Here's how the part is built. I have some questions about the finished solid (model axes, mm). Face numbers are marked on the shaded views. A direction names the side the tool comes from. Give positions to 0.01 mm unless a question says otherwise; leave off trailing zeros. Loops run counter-clockwise (first coordinate to the right, second up) from the corner with the lowest first, then second, coordinate; pieces in that order, holes last.
Q1. If we section it at D-D (z = -11): Please give me the cut outline in (x, y).
Q2. If we section it at B-B (z = 16.5): Please give me the cut outline in (x, y).
Q3. If we section it at A-A (y = 2.8): Please give me the cut outline in (x, z).
Q4. I need wall thicknesses on line 1 (Z direction, x = -33.2, y = 1.7); line 2 (X direction, y = 2.9, z = 0); line 3 (Y direction, x = 14, z = -13). Which ranges of each line are inside material? Lowest first, please.
Q5. If we section it at C-C (x = 8.5): Please give me the cut outline in (y, z).
Q6. We'd pull the mould along X, two halves only. Please class the marked faces 1 and 2: +X half, -X half, draft (parallel to the pull), parting line (faces both ways), or undercut.
Q7. For the marked faces 3 and 4, which set-ups out of +Z, -Z, +X, -X, +Y, -Y let a thin tool reach every point of the face, with its end or its side?
Q8. Will these pins go through, and if not, where does the flat tip stop? P1, Ø0.7, axis at x = -33.2, z = 23, coming from the +Y side; P2, Ø1.4, axis at x = -33.2, z = -24.7, coming from the -Y side; P3, Ø1.3, axis at x = 29.4, z = 19.4, coming from the +Y side (3 decimals).
from build123d import *

# Parameters (mm, degrees)
SKETCH1_W                         = 71
SKETCH1_H                         = 54
BOSS_EXTRUDE1_DEPTH               = 4.15
CUT_EXTRUDE1_DEPTH                = 2
SKETCH4_R                         = 7.5
BOSS_EXTRUDE3_DEPTH               = 2
SKETCH5_R                         = 24
BOSS_EXTRUDE4_DEPTH               = 0.15
M1_4X0_3_TAPPED_HOLE1_D           = 1.1
M1_4X0_3_TAPPED_HOLE1_CSINK_D     = 1.45
M1_4X0_3_TAPPED_HOLE1_CSINK_ANGLE = 90
FILLET1_R                         = 2


with BuildPart() as part:
    # Sketch1 → Boss-Extrude1 (new body)
    with BuildSketch(Plane(origin=(0, 0, 0), x_dir=(1, 0, 0), z_dir=(0, 1, 0))):
        Rectangle(SKETCH1_W, SKETCH1_H)
    extrude(amount=BOSS_EXTRUDE1_DEPTH)

    # Sketch3 → Cut-Extrude1 (cut)
    with BuildSketch(Plane(origin=(0, 4.15, 0), x_dir=(1, 0, 0), z_dir=(0, 1, 0))):
        with BuildLine():
            Line((-6.5, 20), (-33.5, 20))
            Line((-33.5, 20), (-33.5, -19))
            Line((-33.5, -19), (-7.748076809, -19))
            ThreePointArc((-7.748076809, -19), (33.487208249, -0.799639875), (-6.5, 20))
        make_face()
    extrude(amount=-CUT_EXTRUDE1_DEPTH, mode=Mode.SUBTRACT)

    # Sketch4 → Boss-Extrude3 (add)
    with BuildSketch(Plane(origin=(0, 2.15, 0), x_dir=(1, 0, 0), z_dir=(0, 1, 0))):
        with Locations((8.5, 0)):
            Circle(SKETCH4_R)
    extrude(amount=BOSS_EXTRUDE3_DEPTH)

    # Sketch5 → Boss-Extrude4 (add)
    with BuildSketch(Plane(origin=(0, 4.15, 0), x_dir=(1, 0, 0), z_dir=(0, 1, 0))):
        with Locations((8.5, 0)):
            Circle(SKETCH5_R)
    extrude(amount=BOSS_EXTRUDE4_DEPTH)

    # M1.4x0.3 Tapped Hole1 (through all)
    with Locations(Plane(origin=(0, 4.15, 0), x_dir=(1, 0, 0), z_dir=(0, 1, 0))):
        with Locations((-33.2, 24.7), (-33.2, -23), (29.4, -19.4), (32.5, 24.7)):
            CounterSinkHole(M1_4X0_3_TAPPED_HOLE1_D / 2, M1_4X0_3_TAPPED_HOLE1_CSINK_D / 2, counter_sink_angle=M1_4X0_3_TAPPED_HOLE1_CSINK_ANGLE)

    # Fillet1
    fillet1_edges = [part.edges().sort_by_distance(p)[0] for p in [
        (35.5, 2.075, 27),
        (-35.5, 2.075, 27),
        (-35.5, 2.075, -27),
        (35.5, 2.075, -27),
    ]]
    fillet(fillet1_edges, radius=FILLET1_R)


solid = part.part
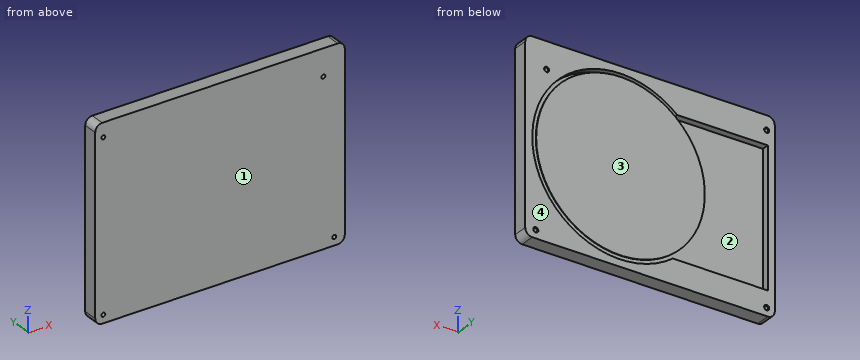
Check sheet entries:
1. outline: (-35.5, 0) - (35.5, 0) - (35.5, 4.15) - (30.95, 4.15) - (30.95, 2.15) - (-33.5, 2.15) - (-33.5, 4.15) - (-35.5, 4.15) - close; (-12.83, 4.15) - (29.83, 4.15) - (29.83, 4.3) - (-12.83, 4.3) - close
2. outline: (-35.5, 0) - (35.5, 0) - (35.5, 4.15) - (27.28, 4.15) - (27.28, 2.15) - (-33.5, 2.15) - (-33.5, 4.15) - (-35.5, 4.15) - close; (-8.93, 4.15) - (25.93, 4.15) - (25.93, 4.3) - (-8.93, 4.3) - close
3. outline: (-35.5, -25) arc R2 ccw to (-33.5, -27) - (33.5, -27) arc R2 ccw to (35.5, -25) - (35.5, 25) arc R2 ccw to (33.5, 27) - (-33.5, 27) arc R2 ccw to (-35.5, 25) - close; circle Ø15 at (8.5, 0); hole circle Ø1.1 at (-33.2, -24.7); hole circle Ø1.1 at (-33.2, 23); hole (-33.5, -20) - (-6.5, -20) arc R25 ccw (long way) to (-7.75, 19) - (-33.5, 19) - close; hole circle Ø1.1 at (29.4, 19.4); hole circle Ø1.1 at (32.5, -24.7)
4. line 1: z = -27 to -25.25, -24.15 to 22.45, 23.55 to 27
4. line 2: x = -35.5 to -33.5, 1 to 16, 33.5 to 35.5
4. line 3: y = 0 to 2.15, 4.15 to 4.3
5. outline: (0, -27) - (4.15, -27) - (4.15, -25) - (2.15, -25) - (2.15, -7.5) - (4.15, -7.5) - (4.15, -24) - (4.3, -24) - (4.3, 24) - (4.15, 24) - (4.15, 7.5) - (2.15, 7.5) - (2.15, 25) - (4.15, 25) - (4.15, 27) - (0, 27) - close
6. face 1: draft
6. face 2: undercut
7. face 3: +Z, -Z, +X, -X, +Y
7. face 4: +Y
8. P1: passes through
8. P2: stops at y = 0
8. P3: stops at y = 4.075
